from build123d import *

# Parameters (mm, degrees)
BOSS_EXTRUDE1_DEPTH = 3.175
SKETCH2_W           = 139.682423128
SKETCH2_H           = 6.35
CUT_EXTRUDE1_DEPTH  = 4.175


with BuildPart() as part:
    # Sketch1 → Boss-Extrude1 (new body)
    with BuildSketch(Plane.XY):
        with BuildLine():
            Line((76.2, 0), (79.375, 0))
            Line((79.375, 0), (79.375, -6.35))
            Line((79.375, -6.35), (-79.375, -6.35))
            Line((-79.375, -6.35), (-79.375, 0))
            Line((-79.375, 0), (-76.2, 0))
            ThreePointArc((-76.2, 0), (0, 76.2), (76.2, 0))
        make_face()
        with BuildLine():
            Line((-69.85, 0), (69.85, 0))
            ThreePointArc((69.85, 0), (0, 69.85), (-69.85, 0))
        make_face(mode=Mode.SUBTRACT)
    extrude(amount=BOSS_EXTRUDE1_DEPTH)

    # Sketch2 → Cut-Extrude1 (cut, through all)
    with BuildSketch(Plane.XY.offset(3.175)):
        with Locations((-0.008788436, -3.175)):
            Rectangle(SKETCH2_W, SKETCH2_H)
    extrude(amount=-CUT_EXTRUDE1_DEPTH, mode=Mode.SUBTRACT)


solid = part.part
Could you check a few things on this model? Use its own coordinates, in mm. A direction names the side the tool comes from. Round coordinates to 2 decimals unless told otherwise and drop trailing zeros. Write each loop counter-clockwise with the first axis right and the second up, starting at its lowest first coordinate (ties: lowest second). Pieces come first, ordered by that corner, then holes. Notation, with made-up numbers: (-23.5, 0.25) -> (-19.5, 0.25) arc R21 cw to (-19.5, 27.25) -> close; hole circle Ø5 at (-23.5, 36). An arc over 180 degrees is marked (long way). Use a Markdown table: item, result.
1. If we section it at C-C (y = 59): List the corners of the cut face in (x, z) for me (3 decimals).
Answer key:
| item | result |
|---|---|
| outline | (-48.223, 0) -> (-37.39, 0) -> (-37.39, 3.175) -> (-48.223, 3.175) -> close; (37.39, 0) -> (48.223, 0) -> (48.223, 3.175) -> (37.39, 3.175) -> close |
2. Please list where these lines run through material, in increasing order: probe 1 along X at (y, z) = (-1.5, 2.4) (3 decimals); probe 2 along X at (y, z) = (29, 3); probe 3 along Y at (x, z) = (4, 1.2).
Answer key:
| item | result |
|---|---|
| probe 1 | x = -79.375 to -69.85, 69.832 to 79.375 |
| probe 2 | x = -70.47 to -63.55, 63.55 to 70.47 |
| probe 3 | y = 69.74 to 76.09 |
3. Which directions (+Z, -Z, +X, -X, +Y, -Y) give clear straight access to the entire face, cutting with the end or side of a thin tool? Please do faces 1 (the face through (-79.375, -3, 2)), 2 (the face through (69.832, -3, 2)), 3 (the face through (-78, 0, 2)), 4 (the face through (78, 0, 2)).
Answer key:
| item | result |
|---|---|
| face 1 | +Z, -Z, -X, +Y, -Y |
| face 2 | +Z, -Z, -Y |
| face 3 | +Z, -Z, -X, +Y |
| face 4 | +Z, -Z, +X, +Y |
4. If we section it at D-D (x = 46.5): List the corners of the cut face in (y, z) for me (3 decimals), then the cut area to 3 significant figures.
Answer key:
| item | result |
|---|---|
| outline | (52.123, 0) -> (60.367, 0) -> (60.367, 3.175) -> (52.123, 3.175) -> close |
| area | 26.2 mm^2 |
5. If we section it at B-B (x = 0): List the corners of the cut face in (y, z) for me (3 decimals).
Answer key:
| item | result |
|---|---|
| outline | (69.85, 0) -> (76.2, 0) -> (76.2, 3.175) -> (69.85, 3.175) -> close |
6. We'd pull the mould along X, two halves only. Please class faces 5 (the face through (-75, -6.35, 2)), 6 (the face through (79.375, -3, 2)), 7 (the face through (-69.85, -3, 2)): +X half, -X half, draft (parallel to the pull), parting line (faces both ways), or undercut.
Answer key:
| item | result |
|---|---|
| face 5 | draft |
| face 6 | +X half |
| face 7 | undercut |
7. If we section it at A-A (y = 13.5): List the corners of the cut face in (x, z) for me (3 decimals), then the cut area to 3 significant figures.
Answer key:
| item | result |
|---|---|
| outline | (-74.995, 0) -> (-68.533, 0) -> (-68.533, 3.175) -> (-74.995, 3.175) -> close; (68.533, 0) -> (74.995, 0) -> (74.995, 3.175) -> (68.533, 3.175) -> close |
| area | 41.0 mm^2 |
8. For pin 1 Ø1 at (x, z) = (78, 1.5) entering from +Y; pin 2 Ø1 at (x, z) = (-25, 0.5) entering from -Y; pin 3 Ø1 at (x, z) = (49.5, 2) entering from +Y, each with a flat end and sliding along its axis, tell me the tip position at first contact or that it passes through.
Answer key:
| item | result |
|---|---|
| pin 1 | stops at y = 0 |
| pin 2 | stops at y = 65.03 |
| pin 3 | stops at y = 58.36 |
